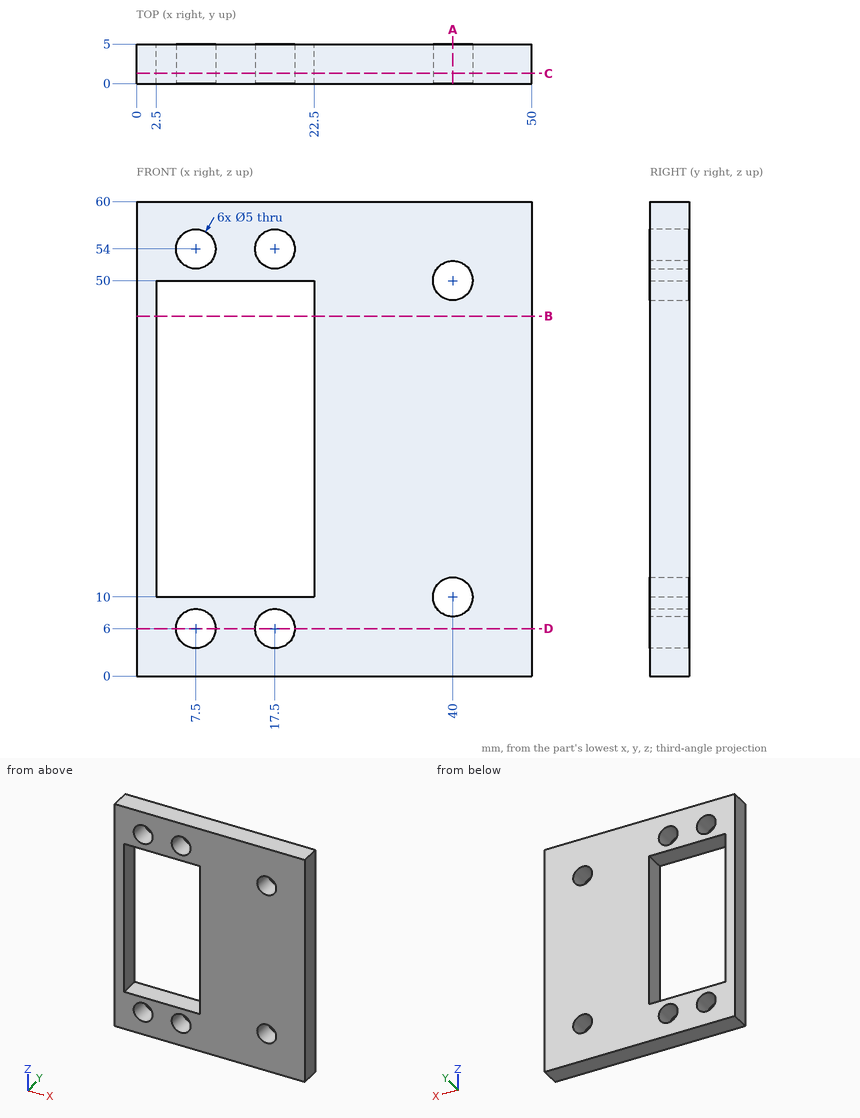
Geometry check sheet. Reference: drawing and pictorial views, mm from the part's lowest x, y, z. Give positions to 0.01 mm unless a question says otherwise; leave off trailing zeros. Loops run counter-clockwise (first coordinate to the right, second up) from the corner with the lowest first, then second, coordinate; pieces in that order, holes last. Notation, with made-up numbers: (1, -2.5) -> (10, -2.5) arc R28 ccw to (10, 36.5) -> close; hole circle Ø3 at (14.5, 64). An arc over 180 degrees is marked (long way). Answer in a Markdown table with one row per item. Add a question column.
1) Cross-section at B-B on z = 45.5. Record the boundary of the cut face in (x, y), and give its area (3 significant figures).
2) Cross-section at A-A on x = 40. Record the boundary of the cut face in (y, z).
3) Cross-section at D-D on z = 6. Record the boundary of the cut face in (x, y), and give its area (3 significant figures).
4) Cross-section at C-C on y = 1.3. Record the boundary of the cut face in (x, z).
5) Material ranges on probe 1 along X at (y, z) = (2.15, 54); probe 2 along X at (y, z) = (1.25, 49.5); probe 3 along Z at (x, y) = (13.5, 4.6), recorded low to high. Write a range as from..to.
Outcome:
| question | item | result |
|---|---|---|
| 1 | outline | (0, 0) -> (2.5, 0) -> (2.5, 5) -> (0, 5) -> close; (22.5, 0) -> (50, 0) -> (50, 5) -> (22.5, 5) -> close |
| 1 | area | 150 mm^2 |
| 2 | outline | (0, 0) -> (5, 0) -> (5, 7.5) -> (0, 7.5) -> close; (0, 12.5) -> (5, 12.5) -> (5, 47.5) -> (0, 47.5) -> close; (0, 52.5) -> (5, 52.5) -> (5, 60) -> (0, 60) -> close |
| 3 | outline | (0, 0) -> (5, 0) -> (5, 5) -> (0, 5) -> close; (10, 0) -> (15, 0) -> (15, 5) -> (10, 5) -> close; (20, 0) -> (50, 0) -> (50, 5) -> (20, 5) -> close |
| 3 | area | 200 mm^2 |
| 4 | outline | (0, 0) -> (50, 0) -> (50, 60) -> (0, 60) -> close; hole (2.5, 10) -> (22.5, 10) -> (22.5, 50) -> (2.5, 50) -> close; hole circle Ø5 at (7.5, 6); hole circle Ø5 at (7.5, 54); hole circle Ø5 at (17.5, 6); hole circle Ø5 at (17.5, 54); hole circle Ø5 at (40, 10); hole circle Ø5 at (40, 50) |
| 5 | probe 1 | x = 0..5, 10..15, 20..50 |
| 5 | probe 2 | x = 0..2.5, 22.5..37.55, 42.45..50 |
| 5 | probe 3 | z = 0..10, 50..60 |
